from build123d import *

# Parameters (mm, degrees)
F1_DEPTH = 6
F2_W     = 25
F2_H     = 6
F3_DEPTH = 6
F5_DEPTH = 6


with BuildPart() as f1:
    # F0 (on Top) → F1 (new body)
    with BuildSketch(Plane.XY):
        with BuildLine():
            Line((-32, -12.5), (32, -12.5))
            Line((32, -12.5), (32, -6.5))
            Line((32, -6.5), (12, -6.5))
            ThreePointArc((12, -6.5), (5.5, 0), (12, 6.5))
            Line((12, 6.5), (32, 6.5))
            Line((32, 6.5), (32, 12.5))
            Line((32, 12.5), (-32, 12.5))
            Line((-32, 12.5), (-32, -12.5))
        make_face()
    extrude(amount=F1_DEPTH)

    # F2 (on face) → F3 (join)
    with BuildSketch(Plane(origin=(-32, 0, 0), x_dir=(0, -1, 0), z_dir=(-1, 0, 0))):
        with Locations((0, 3)):
            Rectangle(F2_W, F2_H)
        with BuildLine():
            ThreePointArc((12.5, 18), (0, 30.5), (-12.5, 18))
            Line((-12.5, 18), (-6.5, 18))
            ThreePointArc((-6.5, 18), (0, 24.5), (6.5, 18))
            Line((6.5, 18), (12.5, 18))
        make_face()
        with BuildLine():
            Line((-12.5, 18), (-12.5, 6))
            Line((-12.5, 6), (12.5, 6))
            Line((12.5, 6), (12.5, 18))
            Line((12.5, 18), (6.5, 18))
            ThreePointArc((6.5, 18), (0, 11.5), (-6.5, 18))
            Line((-6.5, 18), (-12.5, 18))
        make_face()
    extrude(amount=F3_DEPTH)

    # F4 (on face) → F5 (join)
    with BuildSketch(Plane(origin=(0, 12.5, 0), x_dir=(-1, 0, 0), z_dir=(0, 1, 0))):
        with BuildLine():
            Line((38, -12), (38, 6))
            Line((38, 6), (13, 6))
            Line((13, 6), (13, -12))
            ThreePointArc((13, -12), (25.5, 0.5), (38, -12))
        make_face()
        with BuildLine():
            ThreePointArc((13, -12), (25.5, -24.5), (38, -12))
            Line((38, -12), (32, -12))
            ThreePointArc((32, -12), (25.5, -18.5), (19, -12))
            Line((19, -12), (13, -12))
        make_face()
        with BuildLine():
            Line((32, -12), (38, -12))
            ThreePointArc((38, -12), (25.5, 0.5), (13, -12))
            Line((13, -12), (19, -12))
            ThreePointArc((19, -12), (25.5, -5.5), (32, -12))
        make_face()
    extrude(amount=-F5_DEPTH)


solid = f1.part
Part model, mm, in its own coordinate system. A direction names the side the tool comes from. Coordinates: 2 decimals unless noted, no trailing zeros. Loops run counter-clockwise (first coordinate to the right, second up) from the corner with the lowest first, then second, coordinate; pieces in that order, holes last. Notation, with made-up numbers: M -18.75,10.5 L 30.25,10.5 A16 cw 30.25,33.5 Z; hole C -32,75.25 d7. An arc over 180 degrees is marked long. Use a Markdown table: item, result. Add a question column.
Q1. Cut at D-D (y = 11). Write the cut outline in (x, z).
Q2. Cut at C-C (y = 0.5). Write the cut outline in (x, z), and give its area (3 significant figures).
Q3. Cut at A-A (x = -25.5). Write the cut outline in (y, z).
Q4. Probe L1, parallel to Z at x = -25, y = 7; L2, parallel to X at y = 8.85, z = -12; L3, parallel to Z at x = -33.35, y = 0. List the from-to ranges inside material, lowest first.
Q5. Cut at B-B (z = 15.5). Write the cut outline in (x, y), and give its area (3 significant figures).
Q6. Mould opens along X. For faces 4 (the cylindrical face through (-19, 10, -12)), 5 (the flat face through (32, -10, 3)), 6 (the flat face through (22, 6.5, 3)) say: +X half, -X half, draft (parallel to the pull), parting line (faces both ways), or undercut.
Q7. Pin check, flat tips, straight feed: P1, Ø3, axis at x = -21, y = 8.5, coming from the +Z side; P2, Ø5, axis at x = 24, z = -4.5, coming from the -Y side; P3, Ø10, axis at y = 3.5, z = -9, coming from the +X side; P4, Ø10, axis at y = 8.5, z = 17, coming from the +X side. Stop position of each tip, or through.
Q8. Which spindle directions (+Z, -Z, +X, -X, +Y, -Y) get a long thin tool onto all of the face, cutting with end or side? Do faces 1 (the flat face through (-32, 0, 10)), 2 (the flat face through (-13, 10, -6)), 3 (the flat face through (-31, 6.5, -7)). Say none if no direction does.
Worked out:
| question | item | result |
|---|---|---|
| 1 | outline | M -38,-12 A12.5 ccw -13,-12 L -13,0 L 32,0 L 32,6 L -32,6 L -32,23.94 L -38,23.94 Z; hole C -25.5,-12 d13 |
| 2 | outline | M -38,0 L 5.52,0 L 5.52,6 L -32,6 L -32,11.52 L -38,11.52 Z; M -38,24.48 L -32,24.48 L -32,30.49 L -38,30.49 Z |
| 2 | area | 330 mm2 |
| 3 | outline | M -12.5,0 L 6.5,0 L 6.5,-5.5 L 12.5,-5.5 L 12.5,6 L -12.5,6 Z; M 6.5,-24.5 L 12.5,-24.5 L 12.5,-18.5 L 6.5,-18.5 Z |
| 4 | L1 | z = -24.49 to -18.48, -5.52 to 6 |
| 4 | L2 | x = -38 to -32, -19 to -13 |
| 4 | L3 | z = 0 to 11.5, 24.5 to 30.5 |
| 5 | outline | M -38,-12.5 L -32,-12.5 L -32,-6 L -38,-6 Z; M -38,6 L -32,6 L -32,12.5 L -38,12.5 Z |
| 5 | area | 78.0 mm2 |
| 6 | face 4 | undercut |
| 6 | face 5 | +X half |
| 6 | face 6 | draft |
| 7 | P1 | stops at z = 6 |
| 7 | P2 | passes through |
| 7 | P3 | stops at x = -13 |
| 7 | P4 | stops at x = -32 |
| 8 | face 1 | +Z, +X, +Y, -Y |
| 8 | face 2 | -Z, +X, +Y, -Y |
| 8 | face 3 | -Z, +X, -X, -Y |
